Read the model definition and answer for the solid it produces. Units are mm, in the model's axes. A direction names the side the tool comes from. Round coordinates to 2 decimals unless told otherwise and drop trailing zeros. Order: outer loops, then holes, each group sorted by start corner. A loop starts at its lowest first (then second) coordinate and runs counter-clockwise, first axis right, second up. Notation, with made-up numbers: (24.5, -35.5) -> (39.5, -35.5) arc R14 ccw to (39.5, -8.5) -> close; hole circle Ø4 at (-11.75, 46.25). An arc over 180 degrees is marked (long way). Use a Markdown table: item, result. Add a question column.
1. Consider L1, parallel to Y at x = 27, z = 32.5; L2, parallel to X at y = 8.5, z = 5.5; L3, parallel to Z at x = 2.5, y = 35. Determine where each line is inside the solid, lowest interval first. Write a range as [from, to].
2. Section A-A, the plane x = 11 is taken. Give the vertices of the cut face in (y, z), then the cut area to 3 significant figures.
3. For faces 1 (the face through (1, 27, 0)), 2 (the face through (1.5, 26, 22)), 3 (the face through (19, 1.5, -1)), determine the directions among +Z, -Z, +X, -X, +Y, -Y from which every point of the face is accessible in a straight line to the end or side of a thin tool.
4. Section B-B, the plane z = 18.5 is taken. Give the vertices of the cut face in (x, y).
5. Given pin 1 (10.5 mm diameter, centred on x = 21, y = 29.5, fed in from +Z); pin 2 (3.5 mm diameter, centred on x = 16.5, z = -2, fed in from +Y); pin 3 (1.5 mm diameter, centred on x = 14.5, z = -1.5, fed in from -Y), each flat-ended and moving along its own axis, determine where each tip first touches the part or whether it passes through.
6. The mould has two halves that part along X. Classify faces 4 (the face through (36.5, 26, -1)), 5 (the face through (1.5, 26, -1)), 6 (the face through (19, 51.5, 22)): +X half, -X half, draft (parallel to the pull), parting line (faces both ways), or undercut.
7. Section C-C, the plane y = 49 is taken. Give the vertices of the cut face in (x, z), then the cut area to 3 significant figures.
```python
from build123d import *

# Parameters (mm, degrees)
F0_W     = 35
F0_H     = 50
F1_DEPTH = 3
F0_W_2   = 38
F0_H_2   = 53
F2_DEPTH = 1.6
F3_DEPTH = 43
F4_R     = 1


with BuildPart() as f1:
    # F0 (on Top) → F1 (new body)
    with BuildSketch(Plane.XY):
        with Locations((19, 26.5)):
            Rectangle(F0_W, F0_H)
    extrude(amount=-F1_DEPTH)

    # F0 (on Top) → F2 (join)
    with BuildSketch(Plane.XY):
        with Locations((19, 26.5)):
            Rectangle(F0_W_2, F0_H_2)
        with Locations((19, 26.5)):
            Rectangle(F0_W, F0_H, mode=Mode.SUBTRACT)
        with Locations((19, 26.5)):
            Rectangle(F0_W, F0_H)
    extrude(amount=F2_DEPTH)

    # F0 (on Top) → F3 (join)
    with BuildSketch(Plane.XY):
        with Locations((19, 26.5)):
            Rectangle(F0_W_2, F0_H_2)
        with Locations((19, 26.5)):
            Rectangle(F0_W, F0_H, mode=Mode.SUBTRACT)
    extrude(amount=F3_DEPTH)

    # F4
    f4_edges = [f1.edges().sort_by_distance(p)[0] for p in [
        (36.5, 1.5, -1.5),
        (1.5, 1.5, -1.5),
        (1.5, 51.5, -1.5),
        (36.5, 51.5, -1.5),
        (0, 53, 21.5),
        (38, 53, 21.5),
        (0, 0, 21.5),
        (38, 0, 21.5),
    ]]
    fillet(f4_edges, radius=F4_R)


solid = f1.part
```
Verdict:
| question | item | result |
|---|---|---|
| 1 | L1 | y = [0, 1.5], [51.5, 53] |
| 1 | L2 | x = [0, 1.5], [36.5, 38] |
| 1 | L3 | z = [-3, 1.6] |
| 2 | outline | (0, 0) -> (1.5, 0) -> (1.5, -3) -> (51.5, -3) -> (51.5, 0) -> (53, 0) -> (53, 43) -> (51.5, 43) -> (51.5, 1.6) -> (1.5, 1.6) -> (1.5, 43) -> (0, 43) -> close |
| 2 | area | 359 mm2 |
| 3 | face 1 | -Z |
| 3 | face 2 | +Z |
| 3 | face 3 | -Z, +X, -X, -Y |
| 4 | outline | (0, 1) arc R1 ccw to (1, 0) -> (37, 0) arc R1 ccw to (38, 1) -> (38, 52) arc R1 ccw to (37, 53) -> (1, 53) arc R1 ccw to (0, 52) -> close; hole (1.5, 1.5) -> (36.5, 1.5) -> (36.5, 51.5) -> (1.5, 51.5) -> close |
| 5 | pin 1 | stops at z = 1.6 |
| 5 | pin 2 | stops at y = 51.5 |
| 5 | pin 3 | stops at y = 1.5 |
| 6 | face 4 | +X half |
| 6 | face 5 | -X half |
| 6 | face 6 | undercut |
| 7 | outline | (0, 0) -> (1.5, 0) -> (1.5, -3) -> (36.5, -3) -> (36.5, 0) -> (38, 0) -> (38, 43) -> (36.5, 43) -> (36.5, 1.6) -> (1.5, 1.6) -> (1.5, 43) -> (0, 43) -> close |
| 7 | area | 290 mm2 |
